Geometry: final body of the model. Coordinates: model frame, mm. Coordinates: 2 decimals unless noted, no trailing zeros. Write each loop counter-clockwise with the first axis right and the second up, starting at its lowest first coordinate (ties: lowest second). Pieces come first, ordered by that corner, then holes. Notation, with made-up numbers: (-35, 44) -> (0, 44) arc R23 cw to (0, 80) -> close; hole circle Ø1 at (24, 19). An arc over 180 degrees is marked (long way). One line per item, written item: value. Start each with the question number.
from build123d import *

# Parameters (mm, degrees)
CROQUIS1_R              = 6.35
SALIENTE_EXTRUIR1_DEPTH = 3
REDONDEO1_R             = 50
CROQUIS2_R              = 11.5
CORTAR_EXTRUIR1_DEPTH   = 10
CROQUIS6_W              = 3
CROQUIS6_H              = 27
CORTAR_EXTRUIR3_DEPTH   = 4
CROQUIS7_R              = 1.5
CORTAR_EXTRUIR4_DEPTH   = 4
CROQUIS8_R              = 6.5
CORTAR_EXTRUIR5_DEPTH   = 4
CORTAR_EXTRUIR6_DEPTH   = 4


with BuildPart() as part:
    # Croquis1 → Saliente-Extruir1 (new body)
    with BuildSketch(Plane.XY):
        Polygon((-35, 100), (-125, -40), (-125, -100), (125, -100), (125, -40), (35, 100), align=None)
        with Locations((0, 70)):
            Circle(CROQUIS1_R, mode=Mode.SUBTRACT)
    extrude(amount=SALIENTE_EXTRUIR1_DEPTH)

    # Redondeo1
    redondeo1_edges = [part.edges().sort_by_distance(p)[0] for p in [
        (125, -40, 1.5),
        (-125, -40, 1.5),
        (-35, 100, 1.5),
        (35, 100, 1.5),
    ]]
    fillet(redondeo1_edges, radius=REDONDEO1_R)

    # Croquis2 → Cortar-Extruir1 (cut)
    with BuildSketch(Plane.XY.offset(3)):
        with BuildLine():
            ThreePointArc((100, -54.5), (98.5, -53), (97, -54.5))
            Line((97, -54.5), (98.5, -54.5))
            Line((98.5, -54.5), (98.5, -56))
            ThreePointArc((98.5, -56), (99.560660172, -55.560660172), (100, -54.5))
        make_face()
        with BuildLine():
            Line((98.5, -54.5), (97, -54.5))
            ThreePointArc((97, -54.5), (97.439339828, -55.560660172), (98.5, -56))
            Line((98.5, -56), (98.5, -54.5))
        make_face()
        with BuildLine():
            Line((67.5, -56), (67.5, -54.5))
            Line((67.5, -54.5), (69, -54.5))
            ThreePointArc((69, -54.5), (66.439339828, -53.439339828), (67.5, -56))
        make_face()
        with BuildLine():
            Line((69, -54.5), (67.5, -54.5))
            Line((67.5, -54.5), (67.5, -56))
            ThreePointArc((67.5, -56), (68.560660172, -55.560660172), (69, -54.5))
        make_face()
        with Locations((83, -70)):
            Circle(CROQUIS2_R)
        with BuildLine():
            ThreePointArc((69, -85.5), (68.560660172, -84.439339828), (67.5, -84))
            Line((67.5, -84), (67.5, -85.5))
            Line((67.5, -85.5), (69, -85.5))
        make_face()
        with BuildLine():
            Line((67.5, -85.5), (67.5, -84))
            ThreePointArc((67.5, -84), (66.439339828, -86.560660172), (69, -85.5))
            Line((69, -85.5), (67.5, -85.5))
        make_face()
        with BuildLine():
            ThreePointArc((100, -85.5), (99.560660172, -84.439339828), (98.5, -84))
            Line((98.5, -84), (98.5, -85.5))
            Line((98.5, -85.5), (97, -85.5))
            ThreePointArc((97, -85.5), (98.5, -87), (100, -85.5))
        make_face()
        with BuildLine():
            Line((98.5, -85.5), (98.5, -84))
            ThreePointArc((98.5, -84), (97.439339828, -84.439339828), (97, -85.5))
            Line((97, -85.5), (98.5, -85.5))
        make_face()
    extrude(amount=-CORTAR_EXTRUIR1_DEPTH, mode=Mode.SUBTRACT)

    # Croquis6 → Cortar-Extruir3 (cut, through all)
    with BuildSketch(Plane(origin=(0, 0, 0), x_dir=(-1, 0, 0), z_dir=(0, 0, -1))):
        with Locations((-108.5, -86.5)):
            Rectangle(CROQUIS6_W, CROQUIS6_H)
        with Locations((108.5, -86.5)):
            Rectangle(CROQUIS6_W, CROQUIS6_H)
    extrude(amount=-CORTAR_EXTRUIR3_DEPTH, mode=Mode.SUBTRACT)

    # Croquis7 → Cortar-Extruir4 (cut, through all)
    with BuildSketch(Plane(origin=(0, 0, 0), x_dir=(-1, 0, 0), z_dir=(0, 0, -1))):
        with Locations((90, -47)):
            Circle(CROQUIS7_R)
        with Locations((37.6, -52.1)):
            Circle(CROQUIS7_R)
        with Locations((37.6, -80)):
            Circle(CROQUIS7_R)
        with Locations((88.4, -95.3)):
            Circle(CROQUIS7_R)
    extrude(amount=-CORTAR_EXTRUIR4_DEPTH, mode=Mode.SUBTRACT)

    # Croquis8 → Cortar-Extruir5 (cut, through all)
    with BuildSketch(Plane.XY.offset(3)):
        with Locations((-1, -85)):
            Circle(CROQUIS8_R)
        with BuildLine():
            Line((31.5, -88.4), (38.5, -88.4))
            ThreePointArc((38.5, -88.4), (40.1, -90), (38.5, -91.6))
            Line((38.5, -91.6), (31.5, -91.6))
            ThreePointArc((31.5, -91.6), (29.9, -90), (31.5, -88.4))
        make_face()
        with BuildLine():
            Line((31.5, -79.4), (38.5, -79.4))
            ThreePointArc((38.5, -79.4), (40.1, -81), (38.5, -82.6))
            Line((38.5, -82.6), (31.5, -82.6))
            ThreePointArc((31.5, -82.6), (29.9, -81), (31.5, -79.4))
        make_face()
    extrude(amount=-CORTAR_EXTRUIR5_DEPTH, mode=Mode.SUBTRACT)

    # Croquis9 → Cortar-Extruir6 (cut, through all)
    with BuildSketch(Plane(origin=(0, 0, 0), x_dir=(-1, 0, 0), z_dir=(0, 0, -1))):
        with BuildLine():
            Line((-96.95, -49.5), (-96.95, -59.5))
            ThreePointArc((-96.95, -59.5), (-98.5, -61.05), (-100.05, -59.5))
            Line((-100.05, -59.5), (-100.05, -49.5))
            ThreePointArc((-100.05, -49.5), (-98.5, -47.95), (-96.95, -49.5))
        make_face()
        with BuildLine():
            Line((-65.95, -49.5), (-65.95, -59.5))
            ThreePointArc((-65.95, -59.5), (-67.5, -61.05), (-69.05, -59.5))
            Line((-69.05, -59.5), (-69.05, -49.5))
            ThreePointArc((-69.05, -49.5), (-67.5, -47.95), (-65.95, -49.5))
        make_face()
        with BuildLine():
            Line((-69.05, -90.5), (-69.05, -80.5))
            ThreePointArc((-69.05, -80.5), (-67.5, -78.95), (-65.95, -80.5))
            Line((-65.95, -80.5), (-65.95, -90.5))
            ThreePointArc((-65.95, -90.5), (-67.5, -92.05), (-69.05, -90.5))
        make_face()
        with BuildLine():
            Line((-100.05, -90.5), (-100.05, -80.5))
            ThreePointArc((-100.05, -80.5), (-98.5, -78.95), (-96.95, -80.5))
            Line((-96.95, -80.5), (-96.95, -90.5))
            ThreePointArc((-96.95, -90.5), (-98.5, -92.05), (-100.05, -90.5))
        make_face()
    extrude(amount=-CORTAR_EXTRUIR6_DEPTH, mode=Mode.SUBTRACT)


solid = part.part
Q1. Cut plane B-B on x = 83. Output: boundary loops of the cut face in (y, z), and give its area (3 significant figures).
Q2. Cut plane C-C on z = 1.2. Count the separate pieces of the cut face and the enclosed holes in it, and give its area (3 significant figures).
Q3. Cut plane A-A on x = -1. Output: boundary loops of the cut face in (y, z).
Q4. First-contact query: P1, Ø2.5, axis at x = -37.6, y = -52.1, coming from the +Z side; P2, Ø0.9, axis at x = 108.5, z = 2, coming from the -Y side; P3, Ø1.5, axis at y = 34.5, z = 2, coming from the +X side; P4, Ø1, axis at y = 25, z = 1.5, coming from the +X side. Flat tips, straight axial feed; report the tip coordinate or a pass-through.
Q5. Line query: L1, parallel to X at y = -95.3, z = 2.1; L2, parallel to Y at x = -37.6, z = 0.7; L3, parallel to Y at x = 0, z = 2.6. Output: solid intervals per line, ascending. Write a range as from..to.
Q6. Cut plane D-D on y = -32. Output: boundary loops of the cut face in (x, z).
Q7. Draft query along Y for faces 1 (the flat face through (-2, -21, 3)), 2 (the cylindrical face through (-32, 93.7, 1.5)), 3 (the cylindrical face through (-1.38, 63.8, 1.48)), 4 (the cylindrical face through (-2.409, -91.345, 1.521)). Return one class per face: pulls with the +Y half, pulls with the -Y half, needs draft (parallel to the pull), parting line crosses it, or undercut.
Solution:
1. outline: (-100, 0) -> (-81.5, 0) -> (-81.5, 3) -> (-100, 3) -> close; (-58.5, 0) -> (25.33, 0) -> (25.33, 3) -> (-58.5, 3) -> close
1. area: 307 mm²
2. separate pieces: 1
2. enclosed holes: 13
2. area: 36,000 mm²
3. outline: (-100, 0) -> (-91.5, 0) -> (-91.5, 3) -> (-100, 3) -> close; (-78.5, 0) -> (63.73, 0) -> (63.73, 3) -> (-78.5, 3) -> close; (76.27, 0) -> (100, 0) -> (100, 3) -> (76.27, 3) -> close
4. P1: through
4. P2: y = -73
4. P3: x = 77.59
4. P4: x = 83.54
5. L1: -125..-110, -107..-89.9, -86.9..107, 110..125
5. L2: -100..-81.5, -78.5..-53.6, -50.6..90.08
5. L3: -100..-91.42, -78.58..63.65, 76.35..100
6. outline: (-119.56, 0) -> (119.56, 0) -> (119.56, 3) -> (-119.56, 3) -> close
7. face 1: needs draft
7. face 2: pulls with the +Y half
7. face 3: undercut
7. face 4: undercut
